```python
from build123d import *

# Parameters (mm, degrees)
SKETCH1_W                    = 75
SKETCH1_H                    = 16
F_8_0_8_DIAMETER_HOLE1_D     = 8
F_8_0_8_DIAMETER_HOLE1_DEPTH = 30
F_8_0_8_DIAMETER_HOLE1_TIP   = 2.403442476
M6_CLEARANCE_HOLE1_D         = 8
M6_CLEARANCE_HOLE1_DEPTH     = 22
M6_CLEARANCE_HOLE1_TIP       = 2.403442476
SKETCH8_R                    = 17.5
CUT_EXTRUDE1_DEPTH           = 30


with BuildPart() as part:
    # Sketch1 → Revolve1 (revolve)
    with BuildSketch(Plane(origin=(0, 0, 0), x_dir=(1, 0, 0), z_dir=(0, 1, 0))):
        with Locations((37.5, -22)):
            Rectangle(SKETCH1_W, SKETCH1_H)
    revolve(axis=Axis((0, 0, 14), (0, 0, 1)))

    # Ø8.0 (8) Diameter Hole1
    with Locations(Plane(origin=(0, 0, 14), x_dir=(-1, 0, 0), z_dir=(0, 0, -1))):
        with Locations((45.254833996, 45.254833996), (-45.254833996, 45.254833996), (-45.254833996, -45.254833996), (45.254833996, -45.254833996)):
            Hole(F_8_0_8_DIAMETER_HOLE1_D / 2, depth=F_8_0_8_DIAMETER_HOLE1_DEPTH)
            with Locations((0, 0, -(F_8_0_8_DIAMETER_HOLE1_DEPTH + F_8_0_8_DIAMETER_HOLE1_TIP / 2))):  # 118° drill point
                Cone(0, F_8_0_8_DIAMETER_HOLE1_D / 2, F_8_0_8_DIAMETER_HOLE1_TIP, mode=Mode.SUBTRACT)

    # M6 Clearance Hole1
    with Locations(Plane.XY.offset(30)):
        with Locations((0, 64), (0, -64), (64, 0), (-64, 0)):
            Hole(M6_CLEARANCE_HOLE1_D / 2, depth=M6_CLEARANCE_HOLE1_DEPTH)
            with Locations((0, 0, -(M6_CLEARANCE_HOLE1_DEPTH + M6_CLEARANCE_HOLE1_TIP / 2))):  # 118° drill point
                Cone(0, M6_CLEARANCE_HOLE1_D / 2, M6_CLEARANCE_HOLE1_TIP, mode=Mode.SUBTRACT)

    # Sketch8 → Cut-Extrude1 (cut)
    with BuildSketch(Plane.XY.offset(30)):
        Circle(SKETCH8_R)
    extrude(amount=-CUT_EXTRUDE1_DEPTH, mode=Mode.SUBTRACT)


solid = part.part
```
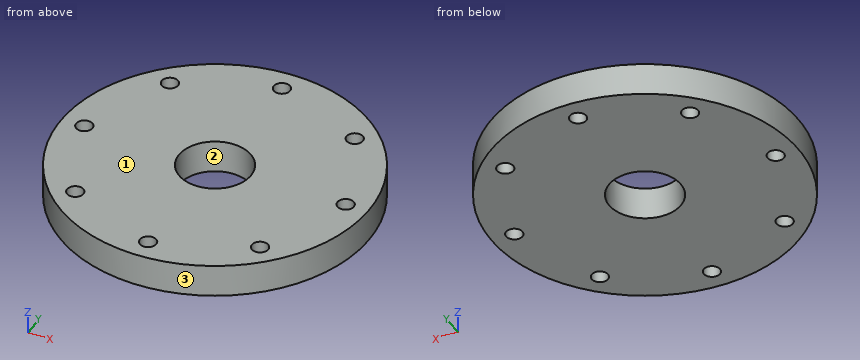
Geometry: final body of the model. Coordinates: model frame, mm. Face numbers are marked on the shaded views. Round coordinates to 2 decimals unless told otherwise and drop trailing zeros. Order: outer loops, then holes, each group sorted by start corner. A loop starts at its lowest first (then second) coordinate and runs counter-clockwise, first axis right, second up. Notation, with made-up numbers: M 71,67.5 L 93,67.5 A23 ccw 93,90.5 Z; hole C 67.25,-20.5 d11. An arc over 180 degrees is marked long. Use one line per item in the form item = value. Start each with the question number.
Q1. Mould query, pull axis X, two halves, no side actions, for the marked faces 1, 2 and 3. Classes: +X half, -X half, draft (parallel to the pull), parting line (faces both ways), or undercut.
Q2. Material intervals for line 1 (Y direction, x = 0, z = 24.25); line 2 (X direction, y = -44.5, z = 25); line 3 (X direction, y = -6, z = 20.5), sorted ascending. Write a range as [from, to].
Q3. Cut plane B-B (x = 64). Return loops of the section in (y, z).
Q4. Cut plane A-A (y = 0). Return loops of the section in (x, z), and give its area (3 significant figures).
Q5. Pin query (flat end, axial travel): pin 1 Ø3 at (y, z) = (19.5, 27) entering from +X; pin 2 Ø6.5 at (x, y) = (-45.25, -45.25) entering from -Z; pin 3 Ø8 at (x, z) = (25, 23) entering from +Y; pin 4 Ø2 at (x, z) = (-31.5, 20.5) entering from -Y. Return the tip coordinate at first contact, or that it passes through.
Geometry results:
q1.face_1 = draft
q1.face_2 = undercut
q1.face_3 = parting line
q2.line_1 = [-75, -68], [-60, -17.5], [17.5, 60], [68, 75]
q2.line_2 = [-60.37, -49.18], [-41.33, 41.33], [49.18, 60.37]
q2.line_3 = [-74.76, -16.44], [16.44, 74.76]
q3.outline = M -39.1,14 L -4,14 L -4,30 L -39.1,30 Z; M 4,14 L 39.1,14 L 39.1,30 L 4,30 Z
q4.outline = M -75,14 L -68,14 L -68,30 L -75,30 Z; M -60,14 L -17.5,14 L -17.5,30 L -60,30 Z; M 17.5,14 L 60,14 L 60,30 L 17.5,30 Z; M 68,14 L 75,14 L 75,30 L 68,30 Z
q4.area = 1,580 mm^2
q5.pin_1 = 72.81
q5.pin_2 = through
q5.pin_3 = 72
q5.pin_4 = -68.52
